Model file for the job. Use its own axes, mm. Face numbers are marked on the shaded views. Round coordinates to 2 decimals unless told otherwise and drop trailing zeros. Order: outer loops, then holes, each group sorted by start corner. A loop starts at its lowest first (then second) coordinate and runs counter-clockwise, first axis right, second up. Notation, with made-up numbers: M 71,70.5 L 94,70.5 A16 cw 94,98.5 Z; hole C 82,-16.75 d6. An arc over 180 degrees is marked long. Return JSON: item names as keys, results as strings. Group by question number.
Item 1: Pin check, flat tips, straight feed: pin 1 Ø0.6 at (y, z) = (-21, 0) entering from -X (3 decimals); pin 2 Ø3 at (y, z) = (12.5, -1) entering from +X (3 decimals); pin 3 Ø3 at (y, z) = (-8.5, 1.5) entering from -X (3 decimals). Stop position of each tip, or through.
Item 2: Slice it at D-D on y = 0. Write the cut outline in (x, z) (3 decimals), then the cut area to 4 significant figures.
Item 3: Slice it at A-A on x = -1.3. Write the cut outline in (y, z), then the cut area to 3 significant figures.
Item 4: Slice it at C-C on y = 22. Write the cut outline in (x, z) (3 decimals).
Item 5: Slice it at B-B on z = 0. Write the cut outline in (x, y) (3 decimals), then the cut area to 4 significant figures.
Item 6: Probe line 1 along Y through (x, z) = (-1.3, -0.75); line 2 along Z through (x, y) = (-0.1, 13.5); line 3 along Z through (x, y) = (-0.2, 0). List the from-to ranges inside material, lowest first.
Item 7: Pull direction Y, two halves, no side cores. Call the marked faces 1, 2 and 3: pulls with the +Y half, pulls with the -Y half, needs draft (parallel to the pull), parting line crosses it, or undercut.
from build123d import *

# Parameters (mm, degrees)
F0_W      = 52
F0_H      = 6.5
F1_DEPTH  = 0.625
F2_W      = 1.25
F2_H      = 6.5
F3_DEPTH  = 1.7
F4_R      = 0.25
F5_R      = 2
F6_DEPTH  = 0.8
F7_W      = 8
F7_H      = 6.5
F8_DEPTH  = 0.3
F9_W      = 6
F9_H      = 3
F10_DEPTH = 0.95
F11_W     = 8.25
F11_H     = 1.25
F12_DEPTH = 0.4


with BuildPart() as f1:
    # F0 (on Right) → F1 (new body, symmetric)
    with BuildSketch(Plane.YZ):
        Rectangle(F0_W, F0_H)
    extrude(amount=F1_DEPTH, both=True)

    # F2 (on face) → F3 (join)
    with BuildSketch(Plane(origin=(-0.625, 0, 0), x_dir=(0, -1, 0), z_dir=(-1, 0, 0))):
        with Locations((-25.375, 0)):
            Rectangle(F2_W, F2_H)
        with Locations((25.375, 0)):
            Rectangle(F2_W, F2_H)
    extrude(amount=F3_DEPTH)

    # F4
    f4_edges = [f1.edges().sort_by_distance(p)[0] for p in [
        (-0.85, -26, 3.25),
        (-0.85, -26, -3.25),
        (-0.85, 26, 3.25),
        (-0.85, 26, -3.25),
    ]]
    fillet(f4_edges, radius=F4_R)

    # F5 (on face) → F6 (cut)
    with BuildSketch(Plane(origin=(-0.625, 0, 0), x_dir=(0, -1, 0), z_dir=(-1, 0, 0))):
        Circle(F5_R)
    extrude(amount=-F6_DEPTH, mode=Mode.SUBTRACT)

    # F7 (on face) → F8 (cut)
    with BuildSketch(Plane.YZ.offset(0.625)):
        with Locations((-13.5, 0)):
            Rectangle(F7_W, F7_H)
        with Locations((13.5, 0)):
            Rectangle(F7_W, F7_H)
    extrude(amount=-F8_DEPTH, mode=Mode.SUBTRACT)

    # F9 (on face) → F10 (cut, through all)
    with BuildSketch(Plane(origin=(-0.625, 0, 0), x_dir=(0, -1, 0), z_dir=(-1, 0, 0))):
        with Locations((13.5, 0)):
            Rectangle(F9_W, F9_H)
        with Locations((-13.5, 0)):
            Rectangle(F9_W, F9_H)
    extrude(amount=-F10_DEPTH, mode=Mode.SUBTRACT)

    # F11 (on face) → F12 (cut)
    with BuildSketch(Plane(origin=(-0.625, 0, 0), x_dir=(0, -1, 0), z_dir=(-1, 0, 0))):
        with Locations((-20.625, 0)):
            Rectangle(F11_W, F11_H)
        with Locations((20.625, 0)):
            Rectangle(F11_W, F11_H)
    extrude(amount=-F12_DEPTH, mode=Mode.SUBTRACT)


solid = f1.part
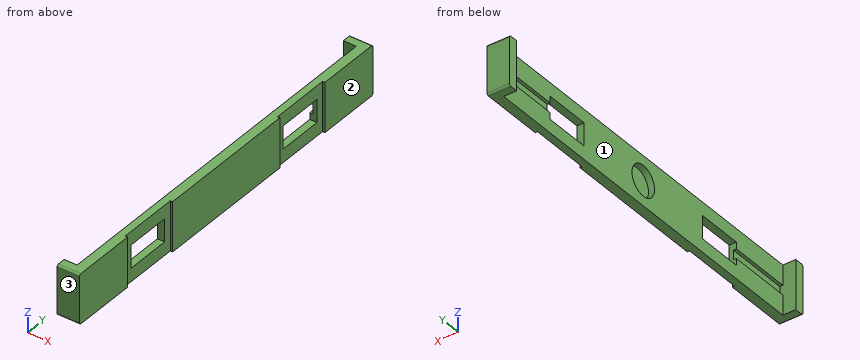
Output values:
{
 "1": {"pin 1": "x = -0.225", "pin 2": "x = 0.325", "pin 3": "x = -0.625"},
 "2": {"outline": "M -0.625,-3.25 L 0.625,-3.25 L 0.625,3.25 L -0.625,3.25 L -0.625,2 L 0.175,2 L 0.175,-2 L -0.625,-2 Z", "area": "4.925 mm²"},
 "3": {"outline": "M -26,-3 A0.25 ccw -25.75,-3.25 L -24.75,-3.25 L -24.75,3.25 L -25.75,3.25 A0.25 ccw -26,3 Z; M 24.75,-3.25 L 25.75,-3.25 A0.25 ccw 26,-3 L 26,3 A0.25 ccw 25.75,3.25 L 24.75,3.25 Z", "area": "16.2 mm²"},
 "4": {"outline": "M -0.625,-3.25 L 0.625,-3.25 L 0.625,3.25 L -0.625,3.25 L -0.625,0.625 L -0.225,0.625 L -0.225,-0.625 L -0.625,-0.625 Z"},
 "5": {"outline": "M -2.325,-26 L 0.625,-26 L 0.625,-17.5 L 0.325,-17.5 L 0.325,-16.5 L -0.225,-16.5 L -0.225,-24.75 L -2.325,-24.75 Z; M -2.325,24.75 L -0.225,24.75 L -0.225,16.5 L 0.325,16.5 L 0.325,17.5 L 0.625,17.5 L 0.625,26 L -2.325,26 Z; M -0.625,-10.5 L 0.325,-10.5 L 0.325,-9.5 L 0.625,-9.5 L 0.625,9.5 L 0.325,9.5 L 0.325,10.5 L -0.625,10.5 L -0.625,2 L 0.175,2 L 0.175,-2 L -0.625,-2 Z", "area": "43.25 mm²"},
 "6": {"line 1": "-26 to -24.75, 24.75 to 26", "line 2": "-3.25 to -1.5, 1.5 to 3.25", "line 3": "-3.25 to -2, 2 to 3.25"},
 "7": {"face 1": "undercut", "face 2": "needs draft", "face 3": "pulls with the -Y half"}
}
